Geometry: final body of the model. Coordinates: model frame, mm. Give positions to 0.01 mm unless a question says otherwise; leave off trailing zeros. Answer in a Markdown table with one row per item. Add a question column.
1) Draft query along X for faces 1 (the conical face through (28.54, -1.1, 9.89)), 2 (the cylindrical face through (28.765, -1.21, 4.807)), 3 (the flat face through (31, 8, 6)), 4 (the flat face through (36.5, 0, 6)). Return one class per face: +X half, -X half, draft (parallel to the pull), parting line (faces both ways), or undercut.
2) First-contact query: P1, Ø5, axis at x = 30.66, y = 0, coming from the +Z side. Flat tip, straight axial feed; report the tip coordinate or a pass-through.
3) Line query: line 1 (X direction, y = 0, z = 5.25) (1 decimal); line 2 (Y direction, x = 30.75, z = 8.5); line 3 (Y direction, x = 28.75, z = 9.5). Output: solid intervals per line, ascending. Write a range as from..to.
Autodesk Inventor part; units mm, degrees
ref_plane "YZ Plane" through (0, 0, 0) normal (1, 0, 0) x (0, 1, 0)
ref_plane "XZ Plane" through (0, 0, 0) normal (0, 1, 0) x (-1, 0, 0)
ref_plane "XY Plane" through (0, 0, 0) normal (0, 0, 1) x (1, 0, 0)
sketch "Sketch1" plane through (0, 0, 0) normal (0, 0, 1) x (1, 0, 0)
  line L0 (23.825, 8.05) -> (23.825, -8.05) construction
  line L1 (37, 8.05) -> (31.3417, 8.05) construction
  line L2 (31.3417, -8.05) -> (37, -8.05) construction
  line L3 (37, 8.05) -> (23.825, 8.05) construction
  line L4 (23.825, 8.05) -> (23.825, -8.05) construction
  line L5 (23.825, -8.05) -> (37, -8.05) construction
  line L6 (37, -8.05) -> (37, 8.05) construction
  circle A0 centre (30.6625, 0) radius 2.067 construction
  line L7 (36.5, -8) -> (24.825, -8)
  line L8 (24.825, -8) -> (24.825, 8)
  line L9 (24.825, 8) -> (36.5, 8)
  line L10 (36.5, 8) -> (36.5, -8)
  line L11 (36.5, -8) -> (24.825, 8) construction
  line L12 (24.825, -8) -> (36.5, 8) construction
  point P0 (0, 0)
  dimension "d0" = 1
  dimension "d1" = 0.05
  dimension "d11" = 11.675
  dimension "d12" = 16
extrude "Extrusion1" add sketch "Sketch1" along normal blind 12
sketch "Sketch2" plane through (0, 0, 12) normal (0, 0, 1) x (1, 0, 0)
  point P0 (0, 0)
  point P1 (30.6625, 0)
hole "Hole1" at (30.6625, 0, 12) direction (0, 0, -1) diameter 4.5 end through all countersink diameter 9 countersink angle 90
properties part number "TH1-002" material "Steel, Mild"
Evaluation:
| question | item | result |
|---|---|---|
| 1 | face 1 | undercut |
| 1 | face 2 | undercut |
| 1 | face 3 | draft |
| 1 | face 4 | +X half |
| 2 | P1 | z = 10 |
| 3 | line 1 | 24.8..28.4, 32.9..36.5 |
| 3 | line 2 | -8..-2.25, 2.25..8 |
| 3 | line 3 | -8..-1.19, 1.19..8 |
